Input: part model. Units: mm. Frame: model coordinates. A direction names the side the tool comes from. Coordinates: 2 decimals unless noted, no trailing zeros. Write each loop counter-clockwise with the first axis right and the second up, starting at its lowest first coordinate (ties: lowest second). Pieces come first, ordered by that corner, then holes. Notation, with made-up numbers: M 66.5,-9.5 L 112.5,-9.5 A11 ccw 112.5,4.5 Z; hole C 23,81 d5. An arc over 180 degrees is marked long. Answer as a JSON object with one key per item and string values. Group by question number.
from build123d import *

# Parameters (mm, degrees)
F1_DEPTH = 24
F0_W     = 8
F0_H     = 8
F2_DEPTH = 16
F3_DEPTH = 8


with BuildPart() as f1:
    # F0 (on Top) → F1 (new body)
    with BuildSketch(Plane.XY):
        Polygon((0, 24), (0, 0), (7, 0), (7, 8), (14, 8), (14, 16), (14, 24), align=None)
    extrude(amount=F1_DEPTH)

    # F0 (on Top) → F2 (join)
    with BuildSketch(Plane.XY):
        with Locations((18, 20)):
            Rectangle(F0_W, F0_H)
    extrude(amount=F2_DEPTH)

    # F0 (on Top) → F3 (join)
    with BuildSketch(Plane.XY):
        with Locations((26, 20)):
            Rectangle(F0_W, F0_H)
    extrude(amount=F3_DEPTH)


solid = f1.part
Q1. Section B-B, the plane z = 6.25. Return the cut outline in (x, y).
Q2. Line query: line 1 (X direction, y = 15, z = 6); line 2 (X direction, y = 2, z = 3.5); line 3 (Y direction, x = 15.25, z = 9.75). Output: solid intervals per line, ascending. Write a range as from..to.
Q3. Access query for faces 1 (the flat face through (26, 20, 8)), 2 (the flat face through (7, 15, 24)), 3 (the flat face through (10, 8, 12)). Directions: +Z, -Z, +X, -X, +Y, -Y. A direction counts if a zero-diameter tool reaches every point of the face in a straight line with its end or side. Return the directions, or none.
Q4. Section C-C, the plane x = 26. Return the cut outline in (y, z).
Q5. Pin query (flat end, axial travel): pin 1 Ø4 at (y, z) = (4.5, 13.5) entering from +X; pin 2 Ø4 at (y, z) = (19.5, 11.5) entering from +X; pin 3 Ø10 at (x, z) = (23, 9.5) entering from -Y. Return the tip coordinate at first contact, or that it passes through.
Q6. Section A-A, the plane y = 22. Return the cut outline in (x, z), and give its area (3 significant figures).
Q7. Section D-D, the plane z = 16.5. Return the cut outline in (x, y), and give its area (3 significant figures).
Filled in:
{
 "1": {"outline": "M 0,0 L 7,0 L 7,8 L 14,8 L 14,16 L 30,16 L 30,24 L 0,24 Z"},
 "2": {"line 1": "0..14", "line 2": "0..7", "line 3": "16..24"},
 "3": {"face 1": "+Z, +X, +Y, -Y", "face 2": "+Z, +X, -X, +Y, -Y", "face 3": "+Z, -Z, +X, -Y"},
 "4": {"outline": "M 16,0 L 24,0 L 24,8 L 16,8 Z"},
 "5": {"pin 1": "x = 7", "pin 2": "x = 22", "pin 3": "y = 16"},
 "6": {"outline": "M 0,0 L 30,0 L 30,8 L 22,8 L 22,16 L 14,16 L 14,24 L 0,24 Z", "area": "528 mm^2"},
 "7": {"outline": "M 0,0 L 7,0 L 7,8 L 14,8 L 14,24 L 0,24 Z", "area": "280 mm^2"}
}
